Print and shaded views of the part. All mm, measured from the part's lowest x, y and z. Round coordinates to 2 decimals unless told otherwise and drop trailing zeros. Order: outer loops, then holes, each group sorted by start corner. A loop starts at its lowest first (then second) coordinate and runs counter-clockwise, first axis right, second up. Notation, with made-up numbers: (83.25, 39.5) -> (113.25, 39.5) arc R7 cw to (113.25, 47.5) -> close; hole circle Ø3 at (-25, 68.5). An arc over 180 degrees is marked (long way). Answer as CSV lines item,"result".
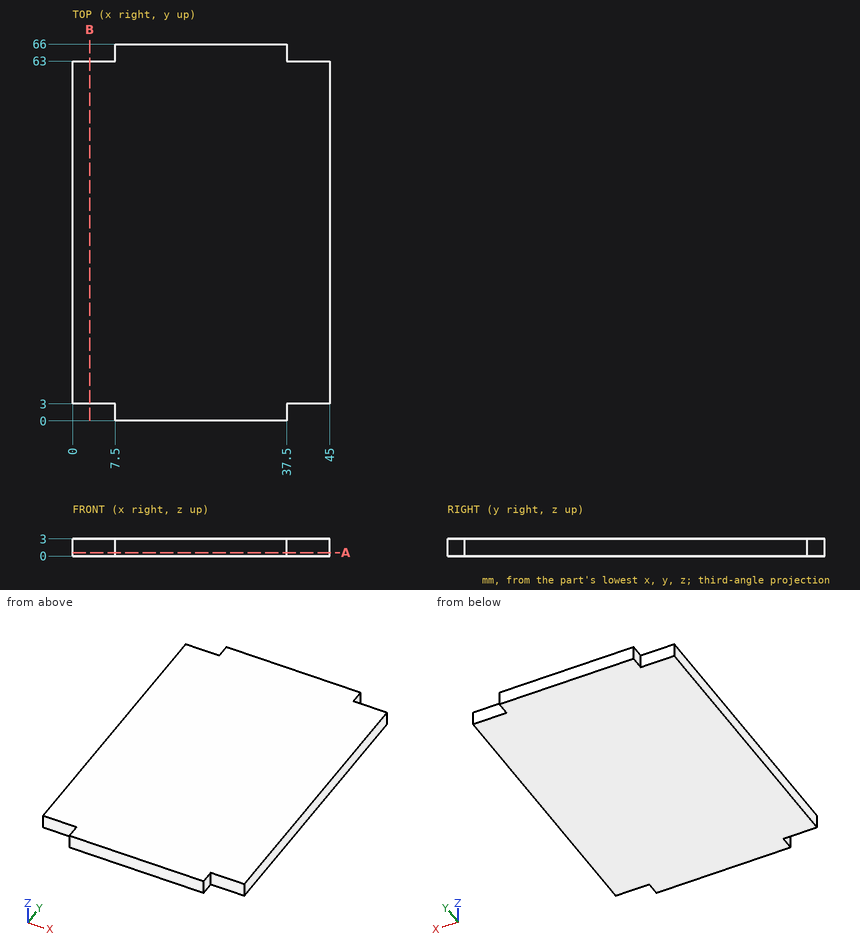
Q1. Saw through at B-B (x = 3). Write the cut outline in (y, z), plus the area to 3 significant figures.
Checks:
outline,"(3, 0) -> (63, 0) -> (63, 3) -> (3, 3) -> close"
area,"180 mm²"
Q2. Flat gauge pins, fed straight in: pin 1 (0.9 mm diameter, centred on y = 1, z = 1.5, fed in from +X); pin 2 (1.5 mm diameter, centred on x = 3.5, z = 2, fed in from -Y); pin 3 (1.5 mm diameter, centred on x = 43, z = 1, fed in from +Y). Where does each tip first touch, or does it go through?
Checks:
pin 1,"x = 37.5"
pin 2,"y = 3"
pin 3,"y = 63"
Q3. Saw through at A-A (z = 0.6). Write the cut outline in (x, y), plus the area to 3 significant figures.
Checks:
outline,"(0, 3) -> (7.5, 3) -> (7.5, 0) -> (37.5, 0) -> (37.5, 3) -> (45, 3) -> (45, 63) -> (37.5, 63) -> (37.5, 66) -> (7.5, 66) -> (7.5, 63) -> (0, 63) -> close"
area,"2,880 mm²"
Q4. Wall check: L1, parallel to Y at x = 41, z = 0.45; L2, parallel to X at y = 63.5, z = 0.3. Give the ranges that are in metal, low to high. Write a range as [from, to].
Checks:
L1,"[3, 63]"
L2,"[7.5, 37.5]"
